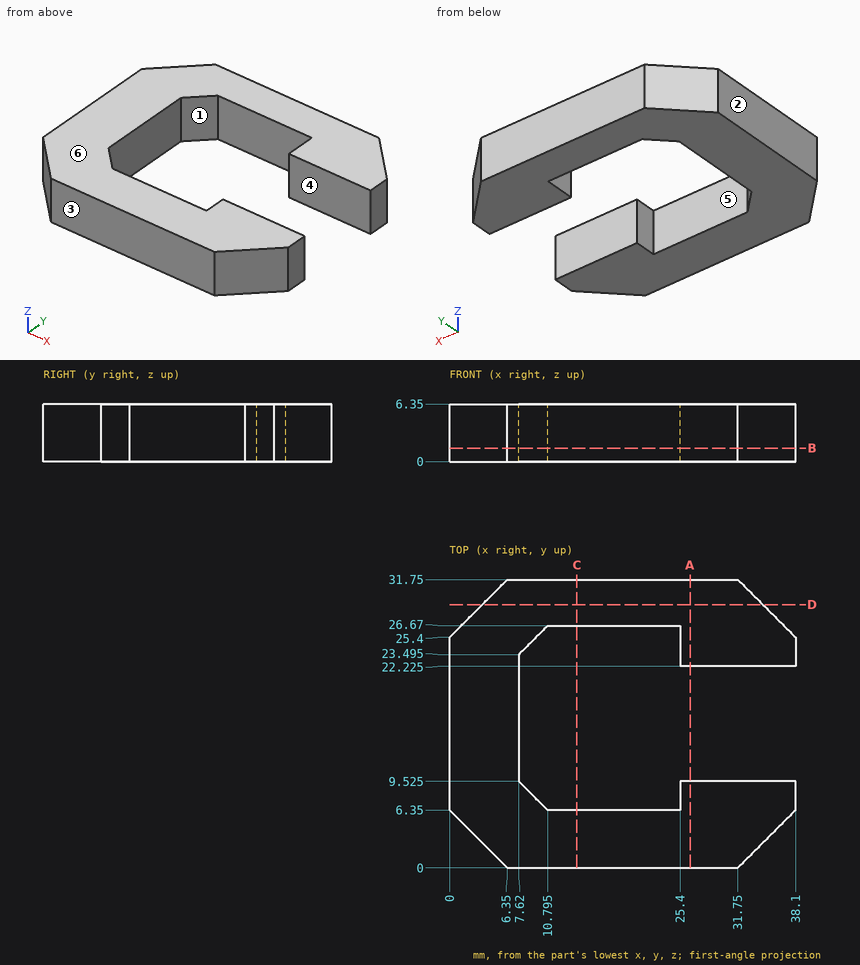
Check sheet for the drawn part. Datum: minimum x, y, z corner. Units: mm. A direction names the side the tool comes from. Give positions to 0.01 mm unless a question says otherwise; leave off trailing zeros. Loops run counter-clockwise (first coordinate to the right, second up) from the corner with the lowest first, then second, coordinate; pieces in that order, holes last.
1) Sectioned sample at D-D, the plane y = 29. Enter the section's corners in (x, z).
2) Draft check along Y on the marked faces 1, 2 and 3. Enter one of: pulls with the +Y half, pulls with the -Y half, needs draft (parallel to the pull), parting line crosses it, or undercut.
3) Sectioned sample at A-A, the plane x = 26.5. Enter the section's corners in (y, z) (3 decimals).
4) Sectioned sample at C-C, the plane x = 14. Enter the section's corners in (y, z).
5) Depth check by flat-ended pin: pin 1 Ø3 at (y, z) = (17, 4.5) entering from +X; pin 2 Ø3 at (x, z) = (33.5, 4) entering from -Y. Enter the tip coordinate at first touch or a pass-through.
6) Thickness scan on line 1 along Y through (x, z) = (23.5, 5); line 2 along X through (y, z) = (22.5, 4.25); line 3 along Y through (x, z) = (30, 6) (3 decimals). Record the ranges inside material, lowest first.
7) Sectioned sample at B-B, the plane z = 1.5. Enter the section's corners in (x, y) (3 decimals), then the cut area to 3 significant figures.
8) Set-up check for the marked faces 4, 5 and 6: record each of +Z, -Z, +X, -X, +Y, -Y from which the full face is reachable in a straight line by a thin tool's end or side.
Answers:
1. outline: (3.6, 0) - (34.5, 0) - (34.5, 6.35) - (3.6, 6.35) - close
2. face 1: undercut
2. face 2: needs draft
2. face 3: pulls with the -Y half
3. outline: (0, 0) - (9.525, 0) - (9.525, 6.35) - (0, 6.35) - close; (22.225, 0) - (31.75, 0) - (31.75, 6.35) - (22.225, 6.35) - close
4. outline: (0, 0) - (6.35, 0) - (6.35, 6.35) - (0, 6.35) - close; (26.67, 0) - (31.75, 0) - (31.75, 6.35) - (26.67, 6.35) - close
5. pin 1: stops at x = 7.62
5. pin 2: stops at y = 0.25
6. line 1: y = 0 to 6.35, 26.67 to 31.75
6. line 2: x = 0 to 7.62, 25.4 to 38.1
6. line 3: y = 0 to 9.525, 22.225 to 31.75
7. outline: (0, 6.35) - (6.35, 0) - (31.75, 0) - (38.1, 6.35) - (38.1, 9.525) - (25.4, 9.525) - (25.4, 6.35) - (10.795, 6.35) - (7.62, 9.525) - (7.62, 23.495) - (10.795, 26.67) - (25.4, 26.67) - (25.4, 22.225) - (38.1, 22.225) - (38.1, 25.4) - (31.75, 31.75) - (6.35, 31.75) - (0, 25.4) - close
7. area: 617 mm2
8. face 4: +Z, -Z, +X
8. face 5: +Z, -Z
8. face 6: +Z, +X, -X, +Y, -Y
